Job drawing, mm, ordinate dimensions from the low corner. One solid piece. Give positions to 0.01 mm unless a question says otherwise; leave off trailing zeros. Order: outer loops, then holes, each group sorted by start corner. A loop starts at its lowest first (then second) coordinate and runs counter-clockwise, first axis right, second up.
1. Drop flat-ended pins along their axis: pin 1 Ø8 at (y, z) = (7, 18) entering from +X (1 decimal); pin 2 Ø8 at (x, z) = (9, 18) entering from +Y (1 decimal); pin 3 Ø1 at (y, z) = (4.5, 28.5) entering from +X. Give the stop position or say it passes through.
2. Slice it at A-A on z = 8. List the corners of the cut face in (x, y) (1 decimal).
3. Probe line 1 (X direction, y = 18, z = 18) (1 decimal); line 2 (Y direction, x = 21.5, z = 16); line 3 (X direction, y = 5, z = 25). List the from-to ranges inside material, lowest first.
4. Slice it at C-C on y = 18. List the corners of the cut face in (x, z) (1 decimal).
5. Slice it at D-D on x = 23.75. List the corners of the cut face in (y, z).
6. Slice it at B-B on x = 5. List the corners of the cut face in (y, z).
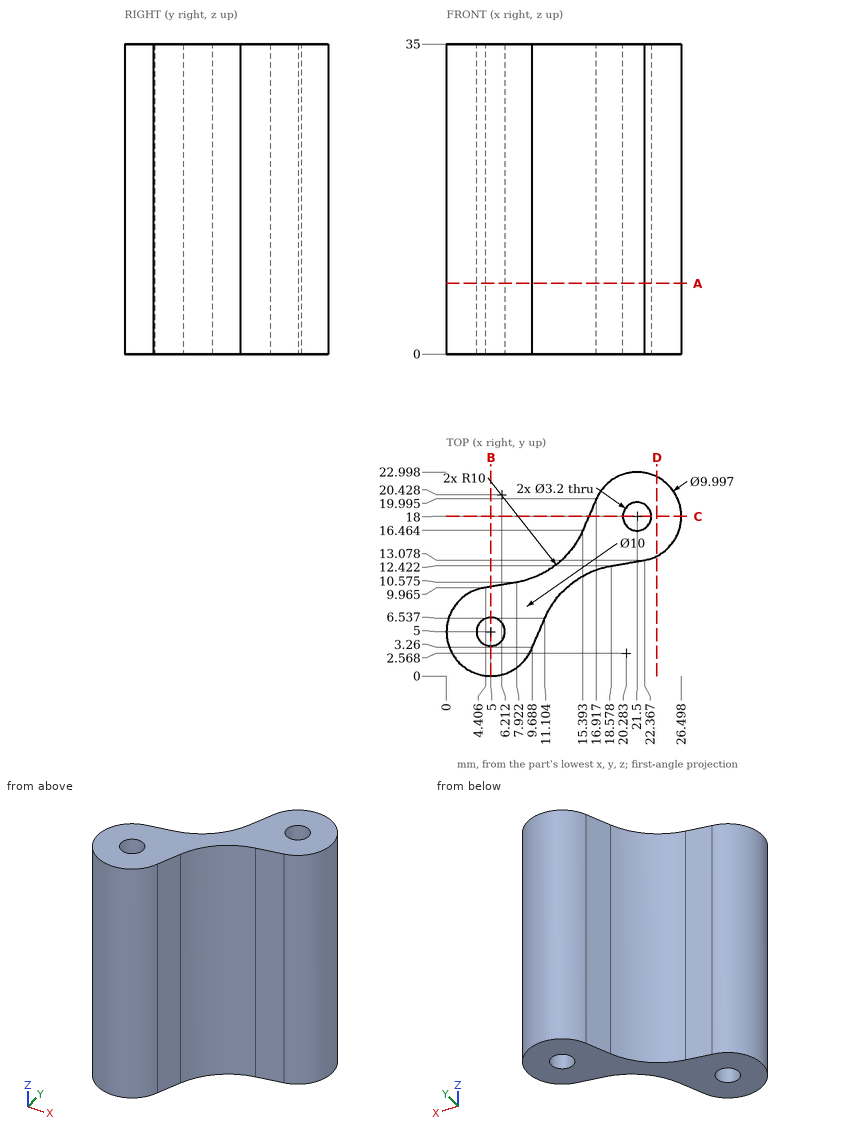
Data:
1. pin 1: stops at x = 14.9
1. pin 2: stops at y = 13.1
1. pin 3: stops at x = 10.44
2. outline: (4.4, 10) arc R5 ccw (long way) to (9.7, 3.3) - (11.1, 6.5) arc R10 cw to (18.6, 12.4) - (22.4, 13.1) arc R5 ccw (long way) to (16.9, 20) - (15.4, 16.5) arc R10 cw to (7.9, 10.6) - close; hole circle Ø3.2 at (5, 5); hole circle Ø3.2 at (21.5, 18)
3. line 1: x = 16.1 to 19.9, 23.1 to 26.5
3. line 2: y = 12.93 to 16.4, 19.6 to 23
3. line 3: x = 0 to 3.4, 6.6 to 10.44
4. outline: (16.1, 0) - (19.9, 0) - (19.9, 35) - (16.1, 35) - close; (23.1, 0) - (26.5, 0) - (26.5, 35) - (23.1, 35) - close
5. outline: (13.54, 0) - (22.46, 0) - (22.46, 35) - (13.54, 35) - close
6. outline: (0, 0) - (3.4, 0) - (3.4, 35) - (0, 35) - close; (6.6, 0) - (10.07, 0) - (10.07, 35) - (6.6, 35) - close
